```python
from build123d import *

# Parameters (mm, degrees)
BOSS_EXTRUDE1_DEPTH = 50
BOSS_EXTRUDE2_START = 1206
SKETCH3_R           = 12.7
BOSS_EXTRUDE2_DEPTH = 1206
BOSS_EXTRUDE3_START = 41
BOSS_EXTRUDE3_DEPTH = 41


with BuildPart() as part:
    # Sketch2 → Boss-Extrude1 (new body)
    with BuildSketch(Plane.XY):
        with BuildLine():
            Line((-17.5, -20.5), (17.5, -20.5))
            Line((17.5, -20.5), (17.5, 20.5))
            ThreePointArc((17.5, 20.5), (0, 26.953663944), (-17.5, 20.5))
            Line((-17.5, 20.5), (-17.5, -20.5))
        make_face()
    extrude(amount=BOSS_EXTRUDE1_DEPTH)

    # Sketch3 → Boss-Extrude2 (add)
    with BuildSketch(Plane(origin=(0, 0, 0), x_dir=(-1, 0, 0), z_dir=(0, 0, -1)).offset(BOSS_EXTRUDE2_START)):
        Circle(SKETCH3_R)
        with BuildLine():
            ThreePointArc((17.5, 20.5), (0, 26.953663944), (-17.5, 20.5))
            Line((-17.5, 20.5), (-17.5, 15.42))
            Line((-17.5, 15.42), (17.5, 15.42))
            Line((17.5, 15.42), (17.5, 20.5))
        make_face()
    extrude(amount=-BOSS_EXTRUDE2_DEPTH)

    # Sketch4 → Boss-Extrude3 (add)
    with BuildSketch(Plane(origin=(0, 0, -1206), x_dir=(-1, 0, 0), z_dir=(0, 0, -1)).offset(BOSS_EXTRUDE3_START)):
        with BuildLine():
            Line((-17.5, 20.5), (-17.5, -20.5))
            Line((-17.5, -20.5), (17.5, -20.5))
            Line((17.5, -20.5), (17.5, 20.5))
            ThreePointArc((17.5, 20.5), (0, 26.953663944), (-17.5, 20.5))
        make_face()
    extrude(amount=-BOSS_EXTRUDE3_DEPTH)


solid = part.part
```
Check sheet for the modelled part. Datum: model origin and axes. Units: mm. A direction names the side the tool comes from. Give positions to 0.01 mm unless a question says otherwise; leave off trailing zeros. Order: outer loops, then holes, each group sorted by start corner. A loop starts at its lowest first (then second) coordinate and runs counter-clockwise, first axis right, second up. Notation, with made-up numbers: (-31, 64.5) -> (18, 64.5) arc R26 cw to (18, 81.5) -> close; hole circle Ø4 at (65.5, 80.5). An arc over 180 degrees is marked (long way). Return JSON: item names as keys, results as strings.
1. Set-up check for faces 5 (the flat face through (8, -10.3, -1206)), 6 (the cylindrical face through (-0.267, 26.952, -607.579)): record each of +Z, -Z, +X, -X, +Y, -Y from which the full face is reachable in a straight line by a thin tool's end or side.
From the geometry:
{"face 5": "none", "face 6": "+Z, -Z, +Y"}
2. Go/stop test with flat-tipped pins: P1, Ø8, axis at x = 3, z = -631.5, coming from the -Y side; P2, Ø3, axis at x = -7, z = -1063, coming from the +Y side; P3, Ø12, axis at y = -10, z = -511, coming from the -X side. Record where each tip stops, or that it passes through.
From the geometry:
{"P1": "y = -12.7", "P2": "y = 26.39", "P3": "x = -12.05"}
3. Mould release check, pull along Z, two halves, no side actions. Record for faces 1 (the flat face through (0, 15.42, -611)), 2 (the flat face through (17.5, 17, -602)), 3 (the flat face through (0, 4, 50)), 4 (the flat face through (0, 4, -1247)): +Z half, -Z half, draft (parallel to the pull), parting line (faces both ways), or undercut.
From the geometry:
{"face 1": "undercut", "face 2": "draft", "face 3": "+Z half", "face 4": "-Z half"}
4. Cross-section at C-C, the plane y = 0. Record the cut outline in (x, z), plus the area to 3 significant figures.
From the geometry:
{"outline": "(-17.5, -1247) -> (17.5, -1247) -> (17.5, -1206) -> (12.7, -1206) -> (12.7, 0) -> (17.5, 0) -> (17.5, 50) -> (-17.5, 50) -> (-17.5, 0) -> (-12.7, 0) -> (-12.7, -1206) -> (-17.5, -1206) -> close", "area": "33,800 mm^2"}
5. Cross-section at A-A, the plane x = 0. Record the cut outline in (y, z).
From the geometry:
{"outline": "(-20.5, -1247) -> (26.95, -1247) -> (26.95, 50) -> (-20.5, 50) -> (-20.5, 0) -> (-12.7, 0) -> (-12.7, -1206) -> (-20.5, -1206) -> close; hole (12.7, -1206) -> (15.42, -1206) -> (15.42, 0) -> (12.7, 0) -> close"}
6. Cross-section at B-B, the plane z = -474. Record the cut outline in (x, y).
From the geometry:
{"outline": "(-17.5, 15.42) -> (17.5, 15.42) -> (17.5, 20.5) arc R26.95 ccw to (-17.5, 20.5) -> close; circle Ø25.4 at (0, 0)"}
7. Material ranges on probe 1 along Y at (x, z) = (0.5, -205.5); probe 2 along Z at (x, y) = (-14.5, 15); probe 3 along X at (y, z) = (2, -1038), recorded low to high. Write a range as [from, to].
From the geometry:
{"probe 1": "[-12.69, 12.69], [15.42, 26.95]", "probe 2": "[-1247, -1206], [0, 50]", "probe 3": "[-12.54, 12.54]"}
